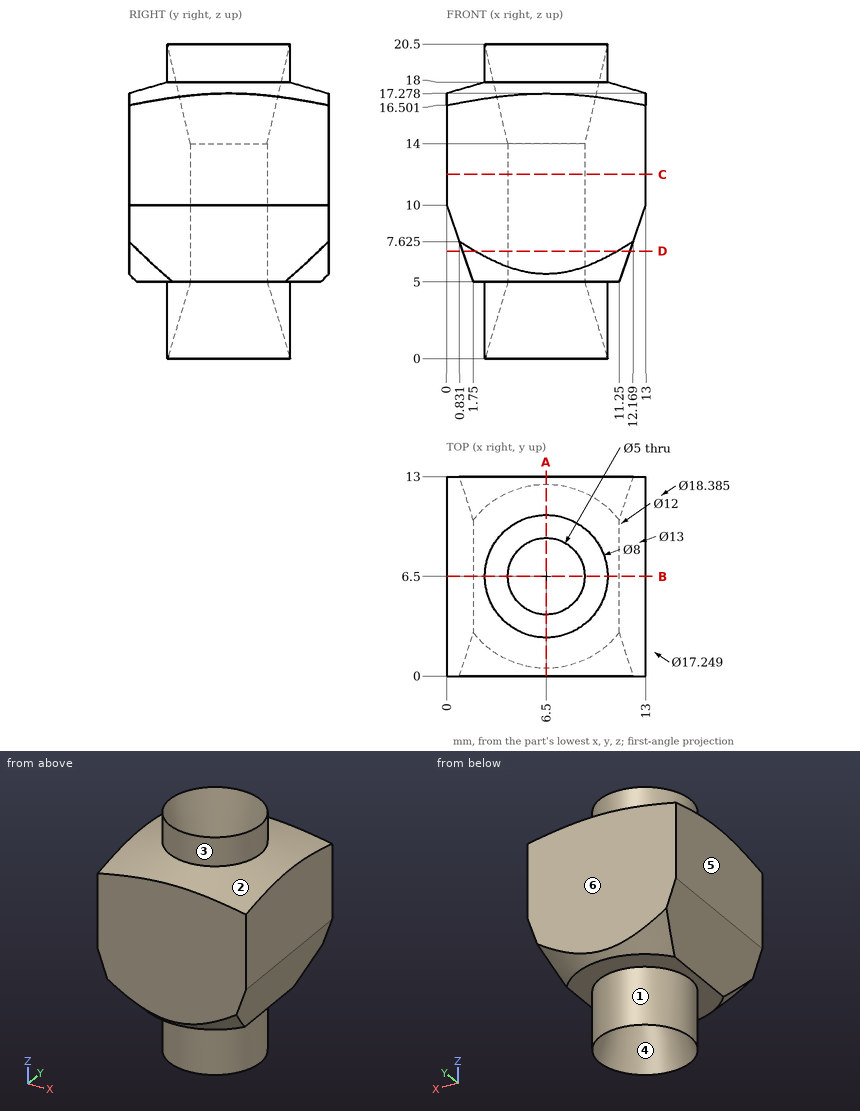
Drawing for the job (mm, zero at the part's lowest x, y, z). A direction names the side the tool comes from. Coordinates: 2 decimals unless noted, no trailing zeros. Loops run counter-clockwise (first coordinate to the right, second up) from the corner with the lowest first, then second, coordinate; pieces in that order, holes last. Notation, with made-up numbers: (-5.5, 52) - (23.5, 52) arc R17 cw to (23.5, 65) - close; hole circle Ø7 at (20.5, 79.5). An arc over 180 degrees is marked (long way). Use CSV: the item, a comma, the result in double quotes. Start each with the question number.
Q1. Drop flat-ended pins along their axis: P1, Ø1.5, axis at x = 10, z = 5, coming from the -Y side; P2, Ø4, axis at y = 1.5, z = 3.5, coming from the +X side; P3, Ø5, axis at x = 4.5, y = 9.5, coming from the -Z side. Give the stop position or say it passes through.
Q2. Cut at D-D, the plane z = 7. List the corners of the cut face in (x, y), then the cut area to 3 significant figures.
Q3. 3-axis set-ups, long thin cutter, end or side, ignore diameter. For the marked faces 1 and 2: which of +Z, -Z, +X, -X, +Y, -Y reach the whole face in a straight line?
Q4. Two-plate mould, pull along Y, no slides. Class the marked faces 3, 4, 5 and 6: +Y half, -Y half, draft (parallel to the pull), parting line (faces both ways), or undercut.
Q5. Cut at A-A, the plane x = 6.5. List the corners of the cut face in (y, z), then the cut area to 3 significant figures.
Q6. Probe probe 1 along Y at (x, z) = (6.5, 10.5); probe 2 along X at (y, z) = (4, 3.25) (1 decimal); probe 3 along Y at (x, z) = (3.25, 19.25) (1 decimal). List the from-to ranges inside material, lowest first. Write a range as from..to.
Q7. Cut at B-B, the plane y = 6.5. List the corners of the cut face in (x, z).
Q8. Cut at C-C, the plane z = 12. List the corners of the cut face in (x, y).
Here are the results:
1,P1,"y = 0.63"
1,P2,"x = 11.28"
1,P3,"z = 0"
2,outline,"(1.05, 0.64) arc R8 ccw to (1.84, 0) - (11.16, 0) arc R8 ccw to (11.95, 0.64) - (11.95, 12.36) arc R8 ccw to (11.16, 13) - (1.84, 13) arc R8 ccw to (1.05, 12.36) - close; hole circle Ø5 at (6.5, 6.5)"
2,area,"121 mm2"
3,face 1,"-Z"
3,face 2,"+Z"
4,face 3,"parting line"
4,face 4,"undercut"
4,face 5,"draft"
4,face 6,"+Y half"
5,outline,"(0, 5.5) - (0.5, 5) - (2.5, 5) - (2.5, 0) - (4, 5) - (4, 14) - (2.5, 20.5) - (2.5, 18) - (0, 17.28) - close; (9, 5) - (10.5, 0) - (10.5, 5) - (12.5, 5) - (13, 5.5) - (13, 17.28) - (10.5, 18) - (10.5, 20.5) - (9, 14) - close"
5,area,"107 mm2"
6,probe 1,"0..4, 9..13"
6,probe 2,"3.4..4.8, 8.2..9.6"
6,probe 3,"4.2..4.7, 8.3..8.8"
7,outline,"(0, 10) - (1.75, 5) - (2.5, 5) - (2.5, 0) - (4, 5) - (4, 14) - (2.5, 20.5) - (2.5, 18) - (0, 17.28) - close; (9, 5) - (10.5, 0) - (10.5, 5) - (11.25, 5) - (13, 10) - (13, 17.28) - (10.5, 18) - (10.5, 20.5) - (9, 14) - close"
8,outline,"(0, 0) - (13, 0) - (13, 13) - (0, 13) - close; hole circle Ø5 at (6.5, 6.5)"
